Geometry: final body of the model. Coordinates: model frame, mm. A direction names the side the tool comes from. Round coordinates to 2 decimals unless told otherwise and drop trailing zeros. Loops run counter-clockwise (first coordinate to the right, second up) from the corner with the lowest first, then second, coordinate; pieces in that order, holes last. Notation, with made-up numbers: (-27, 12.25) - (-3, 12.25) arc R36 cw to (-3, 49.25) - close; hole circle Ø7 at (60, 70.5). An arc over 180 degrees is marked (long way). Write item = value, one per line. Start each with the question number.
Item 1: Line query: line 1 (Y direction, x = 34.85, z = 7.5); line 2 (X direction, y = 36, z = 6); line 3 (Z direction, x = 21.5, y = 23). Output: solid intervals per line, ascending. Write a range as from..to.
Item 2: Draft query along Y for faces 3 (the cylindrical face through (-29.97, 1.32, 7.4)), 4 (the flat face through (-1, 42.5, 478)), 5 (the flat face through (10, 29, 0)). Return one class per face: pulls with the +Y half, pulls with the -Y half, needs draft (parallel to the pull), parting line crosses it, or undercut.
Item 3: Section B-B (y = -24). Return loops of the section in (x, z), plus the area to 3 significant figures.
Item 4: Section C-C (y = 0). Return loops of the section in (x, z), plus the area to 3 significant figures.
Item 5: First-contact query: pin 1 (1 mm diameter, centred on x = -10, y = -16.5, fed in from -Z); pin 2 (8 mm diameter, centred on y = 12, z = 73, fed in from -X). Flat tips, straight axial feed; report the tip coordinate or a pass-through.
Item 6: Access query for faces 1 (the cylindrical face through (-35, 0, 238)), 2 (the flat face through (-1, -42.5, 7)). Directions: +Z, -Z, +X, -X, +Y, -Y. A direction counts if a zero-diameter tool reaches every point of the face in a straight line with its end or side. Return the directions, or none.
Item 7: Section D-D (z = 169.5). Return loops of the section in (x, y).
Item 8: Section A-A (x = 0). Return loops of the section in (y, z), plus the area to 3 significant figures.
from build123d import *

# Parameters (mm, degrees)
CROQUIS1_W              = 97.7
CROQUIS1_H              = 85
CROQUIS1_R              = 3
CROQUIS1_R_2            = 30
SALIENTE_EXTRUIR1_DEPTH = 15
CROQUIS2_R              = 5
SALIENTE_EXTRUIR2_DEPTH = 453
SALIENTE_EXTRUIR3_START = 3
CROQUIS3_W              = 97.7
CROQUIS3_H              = 85
SALIENTE_EXTRUIR3_DEPTH = 20
CHAFL_N1_SIZE           = 1
CHAFL_N2_SIZE           = 1


with BuildPart() as part:
    # Croquis1 → Saliente-Extruir1 (new body)
    with BuildSketch(Plane.XY):
        Rectangle(CROQUIS1_W, CROQUIS1_H)
        with Locations((-34.85, 36.5)):
            Circle(CROQUIS1_R, mode=Mode.SUBTRACT)
        Circle(CROQUIS1_R_2, mode=Mode.SUBTRACT)
        with Locations(Location((34.85, 36.5, 0), (0, 0, 180))):
            Circle(CROQUIS1_R, mode=Mode.SUBTRACT)
        with Locations((34.85, -36.5)):
            Circle(CROQUIS1_R, mode=Mode.SUBTRACT)
        with Locations(Location((-34.85, -36.5, 0), (0, 0, 180))):
            Circle(CROQUIS1_R, mode=Mode.SUBTRACT)
    extrude(amount=SALIENTE_EXTRUIR1_DEPTH)

    # Croquis2 → Saliente-Extruir2 (add)
    with BuildSketch(Plane.XY.offset(15)):
        with Locations(Location((-40, 0, 0), (0, 0, 180))):
            Circle(CROQUIS2_R)
        with Locations(Location((40, 0, 0), (0, 0, 180))):
            Circle(CROQUIS2_R)
    extrude(amount=SALIENTE_EXTRUIR2_DEPTH)

    # Croquis3 → Saliente-Extruir3 (add)
    with BuildSketch(Plane.XY.offset(465).offset(SALIENTE_EXTRUIR3_START)):
        Rectangle(CROQUIS3_W, CROQUIS3_H)
    extrude(amount=SALIENTE_EXTRUIR3_DEPTH)

    # Chaflán1
    chafl_n1_edges = [part.edges().sort_by_distance(p)[0] for p in [
        (48.85, 0, 15),
        (0, 42.5, 15),
        (-48.85, 0, 468),
        (0, 42.5, 468),
        (48.85, 0, 468),
        (-48.85, 0, 15),
    ]]
    chamfer(chafl_n1_edges, length=CHAFL_N1_SIZE)

    # Chaflán2
    chafl_n2_edges = [part.edges().sort_by_distance(p)[0] for p in [
        (48.85, 42.5, 478.5),
        (-48.85, 42.5, 478.5),
        (-48.85, 42.5, 7),
        (48.85, 42.5, 7),
    ]]
    chamfer(chafl_n2_edges, length=CHAFL_N2_SIZE)


solid = part.part
Taken from the geometry:
q1.line_1 = -42.5..-39.5, -33.5..33.5, 39.5..42.5
q1.line_2 = -48.85..-37.81, -31.89..31.89, 37.81..48.85
q1.line_3 = 0..15, 468..488
q2.face_3 = undercut
q2.face_4 = pulls with the +Y half
q2.face_5 = needs draft
q3.outline = (-48.85, 0) - (-18, 0) - (-18, 15) - (-47.85, 15) - (-48.85, 14) - close; (-48.85, 469) - (-47.85, 468) - (47.85, 468) - (48.85, 469) - (48.85, 488) - (-48.85, 488) - close; (18, 0) - (48.85, 0) - (48.85, 14) - (47.85, 15) - (18, 15) - close
q3.area = 2,880 mm^2
q4.outline = (-48.85, 0) - (-30, 0) - (-30, 15) - (-35, 15) - (-35, 468) - (35, 468) - (35, 15) - (30, 15) - (30, 0) - (48.85, 0) - (48.85, 14) - (47.85, 15) - (45, 15) - (45, 468) - (47.85, 468) - (48.85, 469) - (48.85, 488) - (-48.85, 488) - (-48.85, 469) - (-47.85, 468) - (-45, 468) - (-45, 15) - (-47.85, 15) - (-48.85, 14) - close
q4.area = 11,600 mm^2
q5.pin_1 = 468
q5.pin_2 = through
q6.face_1 = none
q6.face_2 = +Z, -Z, +X, -X, -Y
q7.outline = circle Ø10 at (-40, 0); circle Ø10 at (40, 0)
q8.outline = (-42.5, 0) - (-30, 0) - (-30, 15) - (-42.5, 15) - close; (-42.5, 468) - (41.5, 468) - (42.5, 469) - (42.5, 488) - (-42.5, 488) - close; (30, 0) - (42.5, 0) - (42.5, 14) - (41.5, 15) - (30, 15) - close
q8.area = 2,070 mm^2
